```python
from build123d import *

# Parameters (mm, degrees)
SKETCH1_R           = 4
BOSS_EXTRUDE1_DEPTH = 14
SKETCH3_W           = 1
SKETCH3_H           = 11.790173319
CUT_EXTRUDE1_DEPTH  = 19
SKETCH2_R           = 2
CUT_EXTRUDE3_DEPTH  = 31
SKETCH5_R           = 2.75
CUT_EXTRUDE5_DEPTH  = 22


with BuildPart() as part:
    # Sketch1 → Boss-Extrude1 (new body)
    with BuildSketch(Plane.XY):
        Polygon((-21, 0), (21, 0), (21, 6), (9, 6), (9, 32.8), (-9, 32.8), (-9, 6), (-21, 6), align=None)
        with Locations((0, 20)):
            Circle(SKETCH1_R, mode=Mode.SUBTRACT)
    extrude(amount=BOSS_EXTRUDE1_DEPTH)

    # Sketch3 → Cut-Extrude1 (cut)
    with BuildSketch(Plane.XY.offset(14)):
        with Locations((0, 26.904913341)):
            Rectangle(SKETCH3_W, SKETCH3_H)
    extrude(amount=-CUT_EXTRUDE1_DEPTH, mode=Mode.SUBTRACT)

    # Sketch2 → Cut-Extrude3 (cut)
    with BuildSketch(Plane(origin=(9, 0, 0), x_dir=(0, 0, -1), z_dir=(1, 0, 0))):
        with Locations((-7, 28.8)):
            Circle(SKETCH2_R)
    extrude(amount=-CUT_EXTRUDE3_DEPTH, mode=Mode.SUBTRACT)

    # Sketch5 → Cut-Extrude5 (cut)
    with BuildSketch(Plane(origin=(0, 6, 0), x_dir=(1, 0, 0), z_dir=(0, 1, 0))):
        with Locations(Location((16, -7, 0), (0, 0, 180))):
            Circle(SKETCH5_R)
        with Locations(Location((-16, -7, 0), (0, 0, 180))):
            Circle(SKETCH5_R)
    extrude(amount=-CUT_EXTRUDE5_DEPTH, mode=Mode.SUBTRACT)


solid = part.part
```
The model under review builds one solid part; all positions refer to its coordinate system, in mm. A direction names the side the tool comes from. Round coordinates to 2 decimals unless told otherwise and drop trailing zeros. Loops run counter-clockwise (first coordinate to the right, second up) from the corner with the lowest first, then second, coordinate; pieces in that order, holes last. Notation, with made-up numbers: M -21,39.5 L 1,39.5 A27 ccw 1,62.5 Z; hole C -8,38.25 d1. An arc over 180 degrees is marked long. Put each result on its own line as item: value.
Q1. For pin 1 (4.5 mm diameter, centred on y = 27, z = 5.5, fed in from +X); pin 2 (1 mm diameter, centred on y = 18.5, z = 10, fed in from -X); pin 3 (6.5 mm diameter, centred on x = -16, z = 7, fed in from +Y), all flat-tipped, find the tip position at first contact; note any pin that passes through.
Result set:
pin 1: stops at x = 9
pin 2: stops at x = -9
pin 3: stops at y = 6
Q2. Machinability: for faces 1 (the flat face through (-13.6, 6, 5.3)), 2 (the flat face through (9, 19, 7)), 3 (the cylindrical face through (-4.69, 30.783, 7.26)), which of the approach directions +Z, -Z, +X, -X, +Y, -Y give a long, thin tool a straight path to every point of the face, cutting with its end or side? Answer none if there is none.
Result set:
face 1: +Z, -Z, -X, +Y
face 2: +Z, -Z, +X, +Y
face 3: +X, -X
Q3. Consider section C-C, the plane y = 20. Give the boundary of the cut face in (x, z), then the cut area to 3 significant figures.
Result set:
outline: M -9,0 L -4,0 L -4,14 L -9,14 Z; M 4,0 L 9,0 L 9,14 L 4,14 Z
area: 140 mm²
Q4. Consider section D-D, the plane z = 5.5. Give the boundary of the cut face in (x, y), then the cut area to 3 significant figures.
Result set:
outline: M -21,0 L -18.3,0 L -18.3,6 L -21,6 Z; M -13.7,0 L 13.7,0 L 13.7,6 L 9,6 L 9,27.48 L 0.5,27.48 L 0.5,23.97 A4 cw long -0.5,23.97 L -0.5,27.48 L -9,27.48 L -9,6 L -13.7,6 Z; M -9,30.12 L -0.5,30.12 L -0.5,32.8 L -9,32.8 Z; M 0.5,30.12 L 9,30.12 L 9,32.8 L 0.5,32.8 Z; M 18.3,0 L 21,0 L 21,6 L 18.3,6 Z
area: 575 mm²
Q5. To check wall thickness, follow L1, parallel to Z at x = -16, y = 2; L2, parallel to X at y = 26, z = 1.75; L3, parallel to X at y = 20, z = 13.25. State the ranges of each line that lie inside material, in increasing order.
Result set:
L1: z = 0 to 4.25, 9.75 to 14
L2: x = -9 to -0.5, 0.5 to 9
L3: x = -9 to -4, 4 to 9
Q6. Mouldability with a two-part tool opening along X and no side actions: class faces 4 (the flat face through (-21, 3, 7)), 5 (the flat face through (-0.5, 27, 9)), 6 (the flat face through (0, 9, 14)), 7 (the flat face through (0.5, 27, 9)) as released by +X, released by -X, zero draft, split by the parting line, or undercut.
Result set:
face 4: released by -X
face 5: undercut
face 6: zero draft
face 7: undercut
Q7. Consider section B-B, the plane x = 16. Give the boundary of the cut face in (y, z).
Result set:
outline: M 0,0 L 6,0 L 6,4.25 L 0,4.25 Z; M 0,9.75 L 6,9.75 L 6,14 L 0,14 Z
Q8. Consider section A-A, the plane y = 28.8. Give the boundary of the cut face in (x, z), then the cut area to 3 significant figures.
Result set:
outline: M -9,0 L -0.5,0 L -0.5,5 L -9,5 Z; M -9,9 L -0.5,9 L -0.5,14 L -9,14 Z; M 0.5,0 L 9,0 L 9,5 L 0.5,5 Z; M 0.5,9 L 9,9 L 9,14 L 0.5,14 Z
area: 170 mm²
